The listing builds one solid part. Answer for the finished solid, in the listing's coordinates (mm). Face numbers are marked on the shaded views. A direction names the side the tool comes from. Round coordinates to 2 decimals unless told otherwise and drop trailing zeros. Write each loop counter-clockwise with the first axis right and the second up, starting at its lowest first coordinate (ties: lowest second). Pieces come first, ordered by that corner, then holes. Notation, with made-up numbers: (80.5, 62.25) -> (137.5, 62.25) arc R21 ccw to (137.5, 87.25) -> close; hole circle Ø1 at (49, -37.75). An arc over 180 degrees is marked (long way). Write each question's results on one line, items separated by ' | '. Start each with the question number.
```python
from build123d import *

# Parameters (mm, degrees)
F1_DEPTH = 63.5
F2_DEPTH = 25.4
F3_DEPTH = 25.4
F0_W     = 27.3230625695
F0_H     = 23.1139993296
F4_DEPTH = 25.4
F6_R     = 5.08
F7_R     = 5.08
F8_R     = 5.08


with BuildPart() as f1:
    # F0 (on Front) → F1 (new body, symmetric)
    with BuildSketch(Plane.XZ):
        Polygon((62.5374689698, -26.1636357754), (62.5374689698, 26.1636357754), (39.4234696403, 26.1636357754), (-62.5374689698, 26.1636357754), (-62.5374689698, -26.1636357754), align=None)
    extrude(amount=F1_DEPTH, both=True)

    # F0 (on Front) → F2 (join, symmetric)
    with BuildSketch(Plane.XZ):
        with BuildLine():
            Line((39.4234696403, 26.1636357754), (62.5374689698, 26.1636357754))
            Line((62.5374689698, 26.1636357754), (62.5374689698, 58.5364728849))
            ThreePointArc((62.5374689698, 58.5364728849), (69.1652190391, 74.5372769902), (85.1660231445, 81.1650270596))
            Line((85.1660231445, 81.1650270596), (102.0061121875, 81.1650270596))
            Line((102.0061121875, 81.1650270596), (102.0061121875, 104.2790263891))
            Line((102.0061121875, 104.2790263891), (85.1660231445, 104.2790263891))
            ThreePointArc((85.1660231445, 104.2790263891), (52.8211533729, 90.8813426565), (39.4234696403, 58.5364728849))
            Line((39.4234696403, 58.5364728849), (39.4234696403, 26.1636357754))
        make_face()
    extrude(amount=F2_DEPTH, both=True)

    # F0 (on Front) → F3 (join)
    with BuildSketch(Plane.XZ):
        with BuildLine():
            Line((-62.5374689698, 26.1636357754), (39.4234696403, 26.1636357754))
            Line((39.4234696403, 26.1636357754), (39.4234696403, 58.5364728849))
            ThreePointArc((39.4234696403, 58.5364728849), (52.8211533729, 90.8813426565), (85.1660231445, 104.2790263891))
            add(Edge.make_bspline(
                [(-62.5374689698, 26.1636357754), (0, 26.1636357754), (31.0528287573, 104.2790263891), (85.1660231445, 104.2790263891)],
                knots=[0, 0, 0, 0, 167.0878087519, 167.0878087519, 167.0878087519, 167.0878087519], degree=3))
        make_face()
    extrude(amount=F3_DEPTH)

    # F0 (on Front) → F4 (join, symmetric)
    with BuildSketch(Plane.XZ):
        with Locations((115.6676434722, 92.7220267243)):
            Rectangle(F0_W, F0_H)
    extrude(amount=F4_DEPTH, both=True)

    # F0 (on Front) → F5 (revolve)
    with BuildSketch(Plane.XZ):
        Polygon((129.329174757, 104.2790263891), (129.329174757, 81.1650270596), (129.329174757, 75.5129270256), (156.6522373265, 75.5129270256), (156.6522373265, 109.546918422), (129.329174757, 109.546918422), align=None)
    revolve(axis=Axis((129.329174757, 0, 92.5299227238), (0, 0, 1)))

    # F6
    f6_edges = [f1.edges().sort_by_distance(p)[0] for p in [
        (62.537469, -63.5, 0),
    ]]
    fillet(f6_edges, radius=F6_R)

    # F7
    f7_edges = [f1.edges().sort_by_distance(p)[0] for p in [
        (-62.537469, -63.5, 0),
    ]]
    fillet(f7_edges, radius=F7_R)

    # F8
    f8_edges = [f1.edges().sort_by_distance(p)[0] for p in [
        (-62.537469, 63.5, 0),
        (62.537469, 63.5, 0),
    ]]
    fillet(f8_edges, radius=F8_R)


solid = f1.part
```
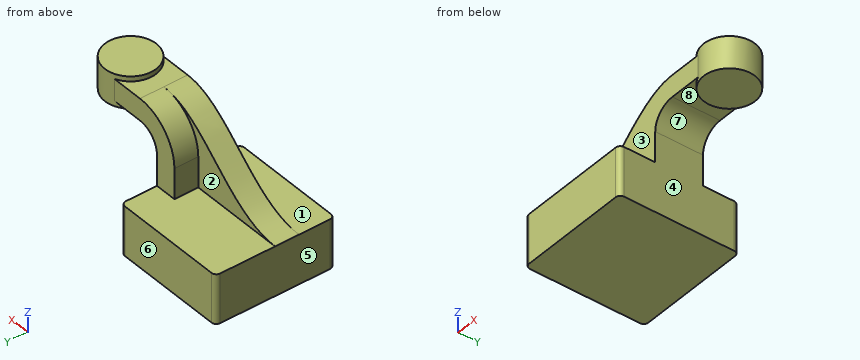
Q1. For the marked faces 1, 2, 3 and 4, determine the directions among +Z, -Z, +X, -X, +Y, -Y from which every point of the face is accessible in a straight line to the end or side of a thin tool.
Q2. The part is cut by section B-B, the plane y = 36. Write down the section's boundary in (x, z).
Q3. Determine the mould class of the marked faces 5, 6, 7 and 8 for opening direction X: pulls with the +X half, pulls with the -X half, needs draft (parallel to the pull), parting line crosses it, or undercut.
Q4. Find the intervals of material crossed by line 1 (Z direction, x = 49.5, y = 52); line 2 (Y direction, x = 55.5, z = 39); line 3 (X direction, y = 9.5, z = 44.5), in increasing order.
Q5. Each of these flat-tipped pins is pushed along its axis until it touches: pin 1 (8 mm diameter, centred on y = 20.5, z = 79.5, fed in from +X); pin 2 (19 mm diameter, centred on x = -1, y = -43.5, fed in from +Z); pin 3 (23.5 mm diameter, centred on x = -6, z = 58.5, fed in from -Y). Where does it stop, or does it pass through?
Q6. The part is cut by section C-C, the plane x = 139. Write down the section's boundary in (y, z), then the cut area to 3 significant figures.
Q7. The part is cut by section A-A, the plane z = -2. Write down the section's boundary in (x, y), then the cut area to 3 significant figures.
Answers follow:
1) face 1: +Z, +X, -X, -Y | face 2: +Z, -X, +Y | face 3: +Z, -X, -Y | face 4: -Z, +X, +Y, -Y
2) outline: (-62.54, -26.16) -> (62.54, -26.16) -> (62.54, 26.16) -> (-62.54, 26.16) -> close
3) face 5: pulls with the -X half | face 6: needs draft | face 7: undercut | face 8: undercut
4) line 1: -26.16 to 26.16 | line 2: -25.4 to 25.4 | line 3: 39.42 to 62.54
5) pin 1: x = 151.11 | pin 2: z = 26.16 | pin 3: y = -25.4
6) outline: (-25.55, 75.51) -> (25.55, 75.51) -> (25.55, 109.55) -> (-25.55, 109.55) -> close | area: 1,740 mm^2
7) outline: (-62.54, -58.42) arc R5.08 ccw to (-57.46, -63.5) -> (57.46, -63.5) arc R5.08 ccw to (62.54, -58.42) -> (62.54, 58.42) arc R5.08 ccw to (57.46, 63.5) -> (-57.46, 63.5) arc R5.08 ccw to (-62.54, 58.42) -> close | area: 15,900 mm^2
